from build123d import *

# Parameters (mm, degrees)
BOSS_EXTRUDE1_DEPTH = 3.5
BOSS_EXTRUDE2_DEPTH = 21
SKETCH3_W           = 23
SKETCH3_H           = 39
BOSS_EXTRUDE3_DEPTH = 2.5
SKETCH5_W           = 21.5
SKETCH5_H           = 25
SKETCH5_W_2         = 7.07
SKETCH5_H_2         = 19.04
BOSS_EXTRUDE5_DEPTH = 2.5
SKETCH6_W           = 7.07
SKETCH6_H           = 5.9
BOSS_EXTRUDE6_DEPTH = 20
BOSS_EXTRUDE7_DEPTH = 23
FILLET1_SIZE        = 10
SKETCH9_R           = 2.475
BOSS_EXTRUDE8_DEPTH = 9
FILLET2_R           = 0.5
SKETCH10_R          = 1.65
CUT_EXTRUDE1_DEPTH  = 9
SKETCH11_W          = 0.2
SKETCH11_H          = 20
CUT_EXTRUDE2_DEPTH  = 9
CUT_EXTRUDE3_DEPTH  = 9
FILLET3_SIZE        = 3
BOSS_EXTRUDE9_DEPTH = 5
SKETCH14_R          = 1.747814763
SKETCH14_R_2        = 1.6
CUT_EXTRUDE4_DEPTH  = 15
SKETCH15_W          = 110
SKETCH15_H          = 3.5
CUT_EXTRUDE5_DEPTH  = 150
FILLET4_SIZE        = 7
FILLET5_SIZE        = 3
FILLET6_SIZE        = 3
SKETCH17_W          = 8
SKETCH17_H          = 21
CUT_EXTRUDE6_DEPTH  = 150
FILLET7_R           = 1
FILLET8_R           = 1
FILLET9_SIZE        = 3


# Some blends are built 0.0001 mm under size
with BuildPart() as part:
    # Sketch1 → Boss-Extrude1 (new body)
    with BuildSketch(Plane(origin=(0, 0, 0), x_dir=(1, 0, 0), z_dir=(0, 1, 0))):
        Polygon((0, 40), (23, 40), (23, 79), (0, 79), (0, 100), (110, 100), (110, 79), (87, 79), (87, 40), (110, 40), (110, 20), (80, 0), (30, 0), (0, 20), align=None)
    extrude(amount=BOSS_EXTRUDE1_DEPTH)

    # Sketch2 → Boss-Extrude2 (add)
    with BuildSketch(Plane(origin=(0, 3.5, 0), x_dir=(1, 0, 0), z_dir=(0, 1, 0))):
        Polygon((0, 79), (23, 79), (23, 40), (0, 40), (0, 37.5), (25.5, 37.5), (25.5, 81.5), (0, 81.5), align=None)
        Polygon((110, 81.5), (84.5, 81.5), (84.5, 37.5), (110, 37.5), (110, 40), (87, 40), (87, 79), (110, 79), align=None)
    extrude(amount=BOSS_EXTRUDE2_DEPTH)

    # Sketch3 → Boss-Extrude3 (add)
    with BuildSketch(Plane(origin=(0, 24.5, 0), x_dir=(1, 0, 0), z_dir=(0, 1, 0))):
        with Locations((11.5, 59.5)):
            Rectangle(SKETCH3_W, SKETCH3_H)
        with Locations((98.5, 59.5)):
            Rectangle(SKETCH3_W, SKETCH3_H)
    extrude(amount=-BOSS_EXTRUDE3_DEPTH)

    # Sketch5 → Boss-Extrude5 (add)
    with BuildSketch(Plane(origin=(0, 24.5, 0), x_dir=(1, 0, 0), z_dir=(0, 1, 0))):
        with Locations((120.75, 50)):
            Rectangle(SKETCH5_W, SKETCH5_H)
        with Locations((-10.75, 50)):
            Rectangle(SKETCH5_W, SKETCH5_H)
        with Locations((29.035, 47.02)):
            Rectangle(SKETCH5_W_2, SKETCH5_H_2)
        with Locations((80.965, 47.02)):
            Rectangle(SKETCH5_W_2, SKETCH5_H_2)
    extrude(amount=-BOSS_EXTRUDE5_DEPTH)

    # Sketch6 → Boss-Extrude6 (add)
    with BuildSketch(Plane(origin=(0, 24.5, 0), x_dir=(1, 0, 0), z_dir=(0, 1, 0))):
        with Locations((29.035, 53.59)):
            Rectangle(SKETCH6_W, SKETCH6_H)
        with Locations((80.965, 53.59)):
            Rectangle(SKETCH6_W, SKETCH6_H)
        with Locations((-17.965, 53.59)):
            Rectangle(SKETCH6_W, SKETCH6_H)
        with Locations((127.965, 53.59)):
            Rectangle(SKETCH6_W, SKETCH6_H)
    extrude(amount=BOSS_EXTRUDE6_DEPTH)

    # Sketch7 → Boss-Extrude7 (add)
    with BuildSketch(Plane(origin=(0, 24.5, 0), x_dir=(1, 0, 0), z_dir=(0, 1, 0))):
        Polygon((0, 81.5), (25.5, 81.5), (25.5, 79), (0, 79), (-21.5, 79), (-21.5, 81.5), align=None)
        Polygon((110, 79), (84.5, 79), (84.5, 81.5), (110, 81.5), (131.5, 81.5), (131.5, 79), align=None)
    extrude(amount=BOSS_EXTRUDE7_DEPTH)

    # Fillet1
    # the kernel refuses this chamfer: 10 mm, written as the material it adds along each edge
    with BuildSketch(Plane(origin=(0, 22, -40), x_dir=(0.027495876610586372, -0.9996219169112968, 0), z_dir=(0, 0, 1)), Plane(origin=(110, 22, -37.5), x_dir=(-0.027495876610586317, -0.9996219169112968, 0), z_dir=(0, 0, -1)), Plane(origin=(110, 24.5, -81.5), x_dir=(0.9996219169112968, 0.027495876610586317, 0), z_dir=(0, 0, 1))) as fillet1_piece_1:
        Polygon((FILLET1_SIZE * 0.999621916911, -FILLET1_SIZE * 0.0274958766106), (-FILLET1_SIZE * 0.0274958766106, -FILLET1_SIZE * 0.999621916911), (0, 0), align=None)
    extrude(amount=2.5)
    with BuildSketch(Plane(origin=(0, 24.5, -79), x_dir=(0.027495876610586372, -0.9996219169112968, 0), z_dir=(0, 0, -1))) as fillet1_piece_2:
        Polygon((FILLET1_SIZE * 0.999621916911, FILLET1_SIZE * 0.0274958766106), (-FILLET1_SIZE * 0.0274958766106, FILLET1_SIZE * 0.999621916911), (0, 0), align=None)
    extrude(amount=2.5)

    # Sketch9 → Boss-Extrude8 (add)
    with BuildSketch(Plane(origin=(0, 0, -81.5), x_dir=(-1, 0, 0), z_dir=(0, 0, -1))):
        with Locations(Location((-114.55, 34.35, 0), (0, 0, 180))):
            Circle(SKETCH9_R)
        with Locations(Location((4.55, 34.35, 0), (0, 0, 180))):
            Circle(SKETCH9_R)
    extrude(amount=BOSS_EXTRUDE8_DEPTH)

    # Fillet2
    fillet2_edges = [part.edges().sort_by_distance(p)[0] for p in [
        (112.075, 34.35, -90.5),
        (-7.025, 34.35, -90.5),
    ]]
    fillet(fillet2_edges, radius=FILLET2_R)

    # Sketch10 → Cut-Extrude1 (cut)
    with BuildSketch(Plane.XY.offset(-50.64)):
        with Locations((129.16, 39.27)):
            Circle(SKETCH10_R)
        with Locations((129.16, 29.43)):
            Circle(SKETCH10_R)
        with Locations((79.77, 39.27)):
            Circle(SKETCH10_R)
        with Locations((79.77, 29.43)):
            Circle(SKETCH10_R)
        with Locations((-19.16, 29.43)):
            Circle(SKETCH10_R)
        with Locations((-19.16, 39.27)):
            Circle(SKETCH10_R)
        with Locations(Location((30.23, 39.27, 0), (0, 0, 180))):
            Circle(SKETCH10_R)
        with Locations(Location((30.23, 29.43, 0), (0, 0, 180))):
            Circle(SKETCH10_R)
    extrude(amount=-CUT_EXTRUDE1_DEPTH, mode=Mode.SUBTRACT)

    # Sketch11 → Cut-Extrude2 (cut)
    with BuildSketch(Plane.XY.offset(-50.64)):
        with Locations((-14.53, 34.5)):
            Rectangle(SKETCH11_W, SKETCH11_H)
        with Locations((25.6, 34.5)):
            Rectangle(SKETCH11_W, SKETCH11_H)
        with Locations((84.4, 34.5)):
            Rectangle(SKETCH11_W, SKETCH11_H)
        with Locations((124.53, 34.5)):
            Rectangle(SKETCH11_W, SKETCH11_H)
    extrude(amount=-CUT_EXTRUDE2_DEPTH, mode=Mode.SUBTRACT)

    # Sketch12 → Cut-Extrude3 (cut)
    with BuildSketch(Plane(origin=(0, 0, -81.5), x_dir=(-1, 0, 0), z_dir=(0, 0, -1))):
        Polygon((-108, 47.5), (-84.5, 25.5), (-84.5, 47.5), align=None)
        Polygon((-25.5, 25.5), (-25.5, 47.5), (-2, 47.5), align=None)
        Polygon((-120, 24.5), (-131.5, 36), (-131.5, 24.5), align=None)
        Polygon((10, 24.5), (21.5, 36), (21.5, 24.5), align=None)
    extrude(amount=-CUT_EXTRUDE3_DEPTH, mode=Mode.SUBTRACT)

    # Fillet3
    fillet3_edges = [part.edges().sort_by_distance(p)[0] for p in [
        (0, 23.25, -62.5),
        (110, 23.25, -62.5),
    ]]
    chamfer(fillet3_edges, length=FILLET3_SIZE)

    # Sketch13 → Boss-Extrude9 (add)
    with BuildSketch(Plane(origin=(0, 3.5, 0), x_dir=(1, 0, 0), z_dir=(0, 1, 0))):
        Polygon((0, 30.5), (32.5, 30.5), (32.5, 88.5), (0, 88.5), (0, 81.5), (25.5, 81.5), (25.5, 37.5), (0, 37.5), align=None)
        Polygon((84.5, 37.5), (110, 37.5), (110, 30.5), (77.5, 30.5), (77.5, 88.5), (110, 88.5), (110, 81.5), (84.5, 81.5), align=None)
    extrude(amount=BOSS_EXTRUDE9_DEPTH)

    # Sketch14 → Cut-Extrude4 (cut)
    with BuildSketch(Plane(origin=(0, 8.5, 0), x_dir=(1, 0, 0), z_dir=(0, 1, 0))):
        with Locations(Location((7.25, 34, 0), (0, 0, 270))):
            Circle(SKETCH14_R)
        with Locations(Location((7.25, 85, 0), (0, 0, 270))):
            Circle(SKETCH14_R_2)
        with Locations(Location((29, 34, 0), (0, 0, 270))):
            Circle(SKETCH14_R_2)
        with Locations(Location((29, 59.5, 0), (0, 0, 270))):
            Circle(SKETCH14_R_2)
        with Locations(Location((29, 85, 0), (0, 0, 270))):
            Circle(SKETCH14_R_2)
        with Locations(Location((81, 34, 0), (0, 0, 90))):
            Circle(SKETCH14_R_2)
        with Locations(Location((102.75, 34, 0), (0, 0, 90))):
            Circle(SKETCH14_R)
        with Locations(Location((81, 59.5, 0), (0, 0, 90))):
            Circle(SKETCH14_R_2)
        with Locations(Location((81, 85, 0), (0, 0, 90))):
            Circle(SKETCH14_R_2)
        with Locations(Location((102.75, 85, 0), (0, 0, 90))):
            Circle(SKETCH14_R_2)
    extrude(amount=-CUT_EXTRUDE4_DEPTH, mode=Mode.SUBTRACT)

    # Sketch15 → Cut-Extrude5 (cut)
    with BuildSketch(Plane(origin=(0, 0, -100), x_dir=(-1, 0, 0), z_dir=(0, 0, -1))):
        Polygon((-77.5, 47.5), (-77.5, 3.5), (0, 3.5), (21.5, 3.5), (21.5, 47.5), align=None)
        with Locations((-55, 1.75)):
            Rectangle(SKETCH15_W, SKETCH15_H)
    extrude(amount=-CUT_EXTRUDE5_DEPTH, mode=Mode.SUBTRACT)

    # Fillet4
    fillet4_edges = [part.edges().sort_by_distance(p)[0] for p in [
        (84.5, 22, -47.02),
    ]]
    chamfer(fillet4_edges, length=FILLET4_SIZE - 0.0001)  # a hair under: the kernel refuses the full size

    # Fillet5
    fillet5_edges = [part.edges().sort_by_distance(p)[0] for p in [
        (87, 22, -59.5),
        (98.5, 22, -79),
        (103.5, 22, -40),
    ]]
    chamfer(fillet5_edges, length=FILLET5_SIZE)

    # Fillet6
    fillet6_edges = [part.edges().sort_by_distance(p)[0] for p in [
        (110, 21.75, -79),
    ]]
    chamfer(fillet6_edges, length=FILLET6_SIZE)

    # Sketch17 → Cut-Extrude6 (cut)
    with BuildSketch(Plane.XZ.offset(-22)):
        with Locations((100, -59.5)):
            Rectangle(SKETCH17_W, SKETCH17_H)
    extrude(amount=-CUT_EXTRUDE6_DEPTH, mode=Mode.SUBTRACT)

    # Fillet7
    fillet7_edges = [part.edges().sort_by_distance(p)[0] for p in [
        (96, 23.25, -70),
        (96, 23.25, -49),
        (104, 23.25, -49),
        (104, 23.25, -70),
    ]]
    fillet(fillet7_edges, radius=FILLET7_R)

    # Fillet8
    fillet8_edges = [part.edges().sort_by_distance(p)[0] for p in [
        (110, 6, -88.5),
        (77.5, 6, -88.5),
        (77.5, 6, -30.5),
        (110, 6, -30.5),
    ]]
    fillet(fillet8_edges, radius=FILLET8_R)

    # Fillet9
    fillet9_edges = [part.edges().sort_by_distance(p)[0] for p in [
        (87, 11.25, -79),
        (87, 11.25, -40),
    ]]
    chamfer(fillet9_edges, length=FILLET9_SIZE)


solid = part.part
Can you work these out from the model? Positions are in its coordinate system, mm. A direction names the side the tool comes from. Coordinates: 2 decimals unless noted, no trailing zeros. Order: outer loops, then holes, each group sorted by start corner. A loop starts at its lowest first (then second) coordinate and runs counter-clockwise, first axis right, second up. Notation, with made-up numbers: M 39.5,43.25 L 75.5,43.25 A15 cw 75.5,61.25 Z; hole C -24,25.5 d8. An arc over 180 degrees is marked long. Write item = value, one per line.
(1) If we mould it in two halves opening along Z, with no side actions, what happens to faces 1 (the face through (81, 34, -50.64)), 2 (the face through (108, 28, -81.5)), 3 (the face through (80.93, 6.04, -83.4)), 4 (the face through (101, 21, -77))? For each: pulls with the +Z half, pulls with the -Z half, needs draft (parallel to the pull), parting line crosses it, or undercut.
Results are:
face_1 = pulls with the +Z half
face_2 = pulls with the -Z half
face_3 = undercut
face_4 = undercut
(2) Suppose I cut it at B-B on x = 129.16. Please give me the cut outline in (y, z).
Results are:
outline = M 22,-62.5 L 24.5,-62.5 L 24.5,-56.54 L 27.78,-56.54 L 27.78,-50.64 L 24.5,-50.64 L 24.5,-37.5 L 22,-37.5 Z; M 31.08,-56.54 L 37.62,-56.54 L 37.62,-50.64 L 31.08,-50.64 Z; M 33.66,-81.5 L 47.5,-81.5 L 47.5,-79 L 33.66,-79 Z; M 40.92,-56.54 L 44.5,-56.54 L 44.5,-50.64 L 40.92,-50.64 Z
(3) I need wall thicknesses on line 1 along Z through (x, y) = (81, 5); line 2 along X through (y, z) = (6, -85); line 3 along Z through (x, y) = (102.75, 7.35). Which ranges of each line are inside material? Lowest first, please. Write a range as [from, to].
Results are:
line_1 = [-88.5, -86.6], [-83.4, -61.1], [-57.9, -35.6], [-32.4, -30.5]
line_2 = [77.5, 79.4], [82.6, 101.15], [104.35, 110]
line_3 = [-88.5, -86.6], [-83.4, -79], [-40, -35.75], [-32.25, -30.5]
(4) Suppose I cut it at C-C on y = 34.35. Please give me the cut outline in (x, z) (3 decimals).
Results are:
outline = M 77.5,-56.54 L 84.3,-56.54 L 84.3,-50.64 L 77.5,-50.64 Z; M 93.953,-81.5 L 112.075,-81.5 L 112.075,-90 A0.5 ccw 112.575,-90.5 L 116.525,-90.5 A0.5 ccw 117.025,-90 L 117.025,-81.5 L 129.85,-81.5 L 129.85,-79 L 93.953,-79 Z; M 124.63,-56.54 L 131.5,-56.54 L 131.5,-50.64 L 124.63,-50.64 Z
(5) For pin 1 Ø5 at (x, y) = (118, 13) entering from -Z; pin 2 Ø8 at (y, z) = (20.5, -80.5) entering from -X; pin 3 Ø1.5 at (x, y) = (114.5, 28.5) entering from -Z; pin 4 Ø8 at (x, y) = (104, 8) entering from -Z, each with a flat end and sliding along its axis, tell me the tip position at first contact or that it passes through.
Results are:
pin_1 = through
pin_2 = 84.5
pin_3 = -81.5
pin_4 = -88.5
(6) Suppose I cut it at D-D on y = 39.27. Please give me the cut outline in (x, z).
Results are:
outline = M 77.5,-56.54 L 78.12,-56.54 L 78.12,-50.64 L 77.5,-50.64 Z; M 81.42,-56.54 L 84.3,-56.54 L 84.3,-50.64 L 81.42,-50.64 Z; M 99.21,-81.5 L 131.5,-81.5 L 131.5,-79 L 99.21,-79 Z; M 124.63,-56.54 L 127.51,-56.54 L 127.51,-50.64 L 124.63,-50.64 Z; M 130.81,-56.54 L 131.5,-56.54 L 131.5,-50.64 L 130.81,-50.64 Z
(7) For faces 5 (the face through (104, 23, -60)), 6 (the face through (81, 18.5, -46.9)), 7 (the face through (128, 44.5, -54)), 8 (the face through (130.734, 39.766, -53.549)), which set-ups out of +Z, -Z, +X, -X, +Y, -Y let a thin tool reach every point of the face, with its end or its side?
Results are:
face_5 = +Y, -Y
face_6 = +Z, -Z, -X
face_7 = +Z, +X, -X, +Y
face_8 = +Z
(8) Suppose I cut it at A-A on x = 122. Please give me the cut outline in (y, z), plus the area to 3 significant figures.
Results are:
outline = M 22,-62.5 L 24.5,-62.5 L 24.5,-37.5 L 22,-37.5 Z; M 26.5,-81.5 L 47.5,-81.5 L 47.5,-79 L 26.5,-79 Z
area = 115 mm2
